Drawing for the job (mm, zero at the part's lowest x, y, z). Round coordinates to 2 decimals unless told otherwise and drop trailing zeros. Write each loop counter-clockwise with the first axis right and the second up, starting at its lowest first coordinate (ties: lowest second). Pieces come first, ordered by that corner, then holes. Notation, with made-up numbers: (67.5, 89.25) -> (96.5, 89.25) arc R20 cw to (96.5, 97.25) -> close; hole circle Ø1 at (55, 14.25). An arc over 180 degrees is marked (long way). One line per question, with ' | ' between items.
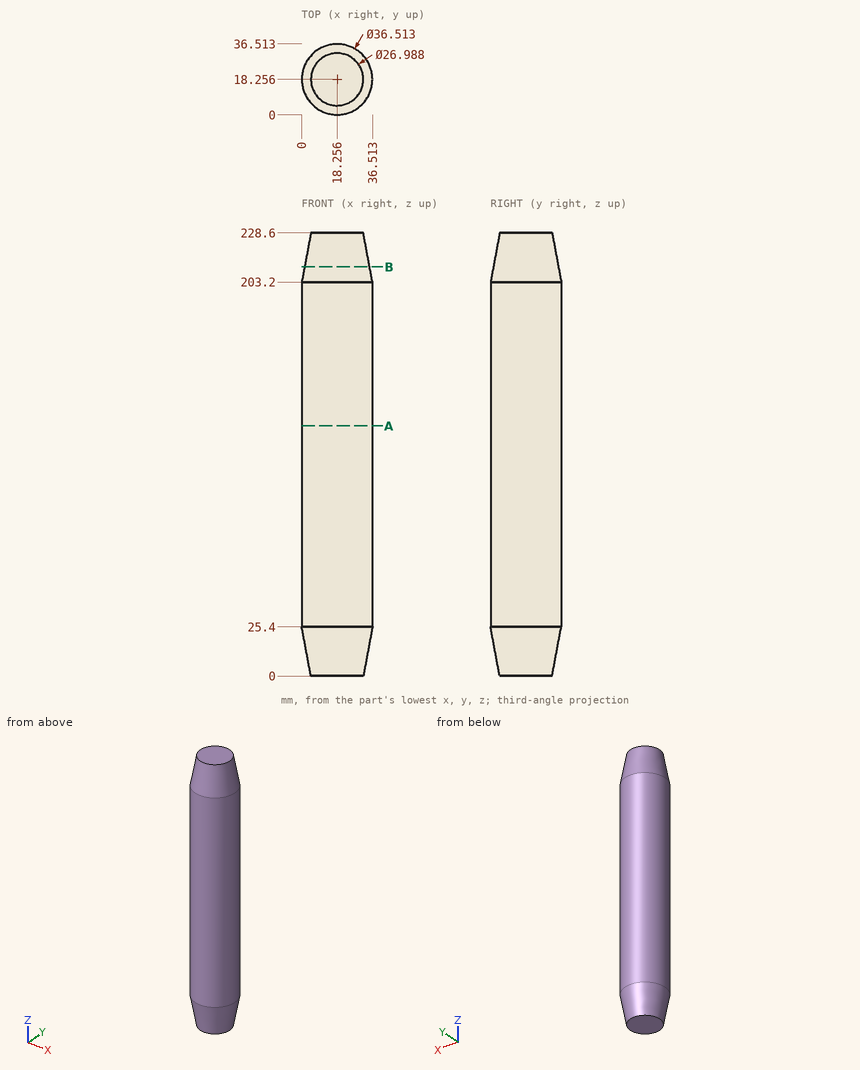
(1) Slice it at A-A (z = 129). Write the cut outline in (x, y).
Calculated:
outline: circle Ø36.51 at (18.26, 18.26)
(2) Slice it at B-B (z = 211). Write the cut outline in (x, y).
Calculated:
outline: circle Ø33.59 at (18.26, 18.26)
(3) Drop flat-ended pins along their axis: pin 1 (3 mm diameter, centred on y = 15, z = 102, fed in from -X) (1 decimal); pin 2 (2 mm diameter, centred on y = 5, z = 51.5, fed in from -X) (1 decimal); pin 3 (6 mm diameter, centred on y = 25, z = 106, fed in from -X). Give the stop position or say it passes through.
Calculated:
pin 1: x = 0.1 | pin 2: x = 4.7 | pin 3: x = 0.39
(4) Wall check: line 1 (Y direction, x = 17, z = 190.5); line 2 (X direction, y = 22, z = 152) (1 decimal); line 3 (Y direction, x = 14, z = 213) (1 decimal). Give the ranges that are in metal, low to high. Write a range as from..to.
Calculated:
line 1: 0.04..36.47 | line 2: 0.4..36.1 | line 3: 2.4..34.1
